```python
from build123d import *

# Parameters (mm, degrees)
SZKIC1_W                        = 10
SZKIC1_H                        = 6.5
DODANIE_WYCI_GNI_CIE1_DEPTH     = 5.5
WYTNIJ_WYCI_GNI_CIE1_REACH      = 28.258
WYTNIJ_WYCI_GNI_CIE1_END_RADIUS = 4.600818815
SZKIC2_W                        = 1
SZKIC2_H                        = 5.5
OTW_R_GWINTOWANY_M3X0_51_D      = 2.5
OTW_R_POD_RUB_M31_REACH         = 34.098
OTW_R_POD_RUB_M31_BORE_R        = 1.6
SZKIC10_R                       = 2.7
WYTNIJ_WYCI_GNI_CIE2_DEPTH      = 24.027157879
ZAOKR_GLENIE1_R                 = 5


with BuildPart() as part:
    # Szkic1 → Dodanie-wyciągnięcie1 (new body)
    with BuildSketch(Plane.XY):
        with BuildLine():
            Line((10, 6.1), (-10, 6.1))
            Line((-10, 6.1), (-10, -3.5))
            Line((-10, -3.5), (-4.583397623, -3.5))
            ThreePointArc((-4.583397623, -3.5), (0, 0.700818815), (4.583397623, -3.5))
            Line((4.583397623, -3.5), (10, -3.5))
            Line((10, -3.5), (10, 6.1))
        make_face()
        with Locations((-15, -6.75)):
            Rectangle(SZKIC1_W, SZKIC1_H)
        with BuildLine():
            Line((-4.583397623, -3.5), (-10, -3.5))
            Line((-10, -3.5), (-10, -10))
            Line((-10, -10), (10, -10))
            Line((10, -10), (10, -3.5))
            Line((10, -3.5), (4.583397623, -3.5))
            ThreePointArc((4.583397623, -3.5), (4.596461454, -3.699810404), (4.600818815, -3.9))
            ThreePointArc((4.600818815, -3.9), (-0.200189596, -8.496461454), (-4.583397623, -3.5))
        make_face()
        with Locations((15, -6.75)):
            Rectangle(SZKIC1_W, SZKIC1_H)
    extrude(amount=DODANIE_WYCI_GNI_CIE1_DEPTH)

    # Wytnij-wyciągnięcie1: up to this cylinder (the profile starts outside it)
    wytnij_wyci_gni_cie1_end = Plane(origin=(0, -3.9, 2.75), z_dir=(0, 0, -1)) * Cylinder(WYTNIJ_WYCI_GNI_CIE1_END_RADIUS, 66.717637631, mode=Mode.PRIVATE)
    # Szkic2 → Wytnij-wyciągnięcie1 (cut, up to the surface)
    with BuildSketch(Plane(origin=(0, 6.1, 0), x_dir=(1, 0, 0), z_dir=(0, 1, 0)), mode=Mode.PRIVATE) as wytnij_wyci_gni_cie1_sk1:
        with Locations((0, -2.75)):
            Rectangle(SZKIC2_W, SZKIC2_H)
    wytnij_wyci_gni_cie1_tool1 = extrude(wytnij_wyci_gni_cie1_sk1.sketch, amount=-WYTNIJ_WYCI_GNI_CIE1_REACH, mode=Mode.PRIVATE) - wytnij_wyci_gni_cie1_end
    add(wytnij_wyci_gni_cie1_tool1.solids().sort_by_distance((0, 6.1, 2.75))[0], mode=Mode.SUBTRACT)

    # Otwór gwintowany M3x0.51 (through all)
    with Locations(Plane(origin=(10, 0, 0), x_dir=(0, 0, -1), z_dir=(1, 0, 0))):
        with Locations((-2.75, 3.38678452)):
            Hole(OTW_R_GWINTOWANY_M3X0_51_D / 2)

    # Otwór pod śrubę M31 bore → Otwór pod śrubę M31 (cut, up to next)
    with BuildSketch(Plane(origin=(10, 0, 0), x_dir=(0, 0, -1), z_dir=(1, 0, 0)), mode=Mode.PRIVATE) as otw_r_pod_rub_m31_sk1:
        with Locations((-2.75, 3.38678452)):
            Circle(OTW_R_POD_RUB_M31_BORE_R)
    otw_r_pod_rub_m31_tool1 = extrude(otw_r_pod_rub_m31_sk1.sketch, amount=-OTW_R_POD_RUB_M31_REACH, mode=Mode.PRIVATE) & part.part
    add(otw_r_pod_rub_m31_tool1.solids().sort_by_distance((10, 3.386785, 2.75))[0], mode=Mode.SUBTRACT)

    # Szkic10 → Wytnij-wyciągnięcie2 (cut, through all)
    with BuildSketch(Plane.XY.offset(5.5)):
        with Locations((8.363131331, -6.679576829)):
            Circle(SZKIC10_R)
    extrude(amount=-WYTNIJ_WYCI_GNI_CIE2_DEPTH, mode=Mode.SUBTRACT)

    # Zaokrąglenie1
    zaokr_glenie1_edges = [part.edges().sort_by_distance(p)[0] for p in [
        (-10, -3.5, 2.75),
        (10, -3.5, 2.75),
    ]]
    fillet(zaokr_glenie1_edges, radius=ZAOKR_GLENIE1_R)


solid = part.part
```
Input: part model. Units: mm. Frame: model coordinates. A direction names the side the tool comes from. Coordinates: 2 decimals unless noted, no trailing zeros. Loops run counter-clockwise (first coordinate to the right, second up) from the corner with the lowest first, then second, coordinate; pieces in that order, holes last. Notation, with made-up numbers: (-29, 62) -> (-21, 62) arc R25 cw to (-21, 82) -> close; hole circle Ø4 at (67.25, 54.25). An arc over 180 degrees is marked (long way). Use a Markdown table: item, result.
1) Cut plane B-B (x = 3). Return the cut outline in (y, z), then the cut area to 3 significant figures.
Results found:
| item | result |
|---|---|
| outline | (-10, 0) -> (-7.39, 0) -> (-7.39, 5.5) -> (-10, 5.5) -> close; (-0.41, 0) -> (6.1, 0) -> (6.1, 5.5) -> (-0.41, 5.5) -> close; hole circle Ø3.2 at (3.39, 2.75) |
| area | 42.1 mm2 |
2) Material intervals for line 1 along X through (y, z) = (-7.25, 3.95); line 2 along X through (y, z) = (1.25, 0.5); line 3 along X through (y, z) = (-5.25, 4.5), sorted ascending. Write a range as from..to.
Results found:
| item | result |
|---|---|
| line 1 | x = -20..-3.15, 3.15..5.72, 11..20 |
| line 2 | x = -10.01..-0.5, 0.5..10.01 |
| line 3 | x = -20..-4.4, 4.4..6.07, 10.65..20 |
3) Cut plane C-C (y = -1). Return the cut outline in (x, z).
Results found:
| item | result |
|---|---|
| outline | (-10.67, 0) -> (-3.57, 0) -> (-3.57, 5.5) -> (-10.67, 5.5) -> close; (3.57, 0) -> (10.67, 0) -> (10.67, 5.5) -> (3.57, 5.5) -> close |
4) Contact query for flat-ended pins moving along their axis: pin 1 (2.5 mm diameter, centred on y = 4.5, z = 3, fed in from -X); pin 2 (2.5 mm diameter, centred on y = 4, z = 3.5, fed in from +X); pin 3 (2 mm diameter, centred on y = 3.39, z = 2.75, fed in from +X); pin 4 (2.5 mm diameter, centred on x = -17, z = 3.5, fed in from +Y). Output: stop coordinate, or through.
Results found:
| item | result |
|---|---|
| pin 1 | stops at x = -10 |
| pin 2 | stops at x = 10 |
| pin 3 | passes through |
| pin 4 | stops at y = -3.5 |
5) Access query for faces 1 (the flat face through (-0.5, 5, 3)), 2 (the flat face through (17, -3.5, 3)), 3 (the flat face through (-18, -3.5, 3)), 4 (the cylindrical face through (5.316, 4.973, 2.958)). Directions: +Z, -Z, +X, -X, +Y, -Y. A direction counts if a zero-diameter tool reaches every point of the face in a straight line with its end or side. Return the directions, or none.
Results found:
| item | result |
|---|---|
| face 1 | +Z, -Z, +Y |
| face 2 | +Z, -Z, +X, +Y |
| face 3 | +Z, -Z, -X, +Y |
| face 4 | +X |
6) Cut plane A-A (z = 2.4). Return the cut outline in (x, y), then the cut area to 3 significant figures.
Results found:
| item | result |
|---|---|
| outline | (-20, -10) -> (20, -10) -> (20, -3.5) -> (15, -3.5) arc R5 cw to (10, 1.5) -> (10, 1.83) -> (0.5, 1.83) -> (0.5, 0.67) arc R4.6 cw (long way) to (-0.5, 0.67) -> (-0.5, 2.19) -> (-10, 2.19) -> (-10, 1.5) arc R5 cw to (-15, -3.5) -> (-20, -3.5) -> close; (-10, 4.59) -> (-0.5, 4.59) -> (-0.5, 6.1) -> (-10, 6.1) -> close; (0.5, 4.95) -> (10, 4.95) -> (10, 6.1) -> (0.5, 6.1) -> close; hole circle Ø5.4 at (8.36, -6.68) |
| area | 315 mm2 |
7) Cut plane D-D (x = -2). Return the cut outline in (y, z).
Results found:
| item | result |
|---|---|
| outline | (-10, 0) -> (-8.04, 0) -> (-8.04, 5.5) -> (-10, 5.5) -> close; (0.24, 0) -> (6.1, 0) -> (6.1, 5.5) -> (0.24, 5.5) -> close; hole circle Ø2.5 at (3.39, 2.75) |
8) Pull-direction query (Z, two-part tool) for faces 5 (the flat face through (-5, -4, 5.5)), 6 (the cylindrical face through (-5.32, 2.28, 3.33)), 7 (the flat face through (20, -7, 3)); classes: released by +Z, released by -Z, zero draft, split by the parting line, or undercut.
Results found:
| item | result |
|---|---|
| face 5 | released by +Z |
| face 6 | undercut |
| face 7 | zero draft |
